Autodesk Inventor part; units mm, degrees
ref_plane "YZ Plane" through (0, 0, 0) normal (1, 0, 0) x (0, 1, 0)
ref_plane "XZ Plane" through (0, 0, 0) normal (0, 1, 0) x (-1, 0, 0)
ref_plane "XY Plane" through (0, 0, 0) normal (0, 0, 1) x (1, 0, 0)
sketch "Szkic1" plane through (0, 0, 0) normal (0, 0, 1) x (1, 0, 0)
  line L0 (-98.62, 58.242) -> (467.38, 58.242)
  line L1 (467.38, 58.242) -> (467.38, -3.758)
  line L2 (467.38, -3.758) -> (-98.62, -3.758)
  line L3 (-98.62, -3.758) -> (-98.62, 58.242)
  line L4 (65.48, 58.242) -> (95.48, 58.242)
  line L5 (95.48, 58.242) -> (95.48, 86.242)
  line L6 (95.48, 86.242) -> (65.48, 86.242)
  line L7 (65.48, 86.242) -> (65.48, 58.242)
  line L8 (258.28, 58.242) -> (288.28, 58.242)
  line L9 (288.28, 58.242) -> (288.28, 86.242)
  line L10 (288.28, 86.242) -> (258.28, 86.242)
  line L11 (258.28, 86.242) -> (258.28, 58.242)
  line L12 (-98.62, 58.242) -> (-98.62, 88.242)
  line L13 (-98.62, 88.242) -> (-68.62, 88.242)
  line L14 (-68.62, 88.242) -> (-68.62, 58.242)
  line L15 (-28.62, 50.242) -> (21.38, 50.242)
  line L16 (21.38, 50.242) -> (21.38, 0.242)
  line L17 (21.38, 0.242) -> (-28.62, 0.242)
  line L18 (-28.62, 0.242) -> (-28.62, 50.242)
  circle A0 centre (-23.62, 45.242) radius 1.5
  circle A1 centre (16.38, 45.242) radius 1.5
  circle A2 centre (-23.62, 5.242) radius 1.5
  circle A3 centre (16.38, 5.242) radius 1.5
  circle A4 centre (-3.62, 25.242) radius 24
  circle A5 centre (-3.62, 25.242) radius 11
  arc A6 (9.6779, 5.2628) -> (4.7367, 18.0889) centre (-10.3192, 4.9238) ccw
  arc A7 (12.5064, 7.4673) -> (6.6011, 21.1764) centre (-7.4877, 6.9811) ccw
  arc A8 (19.4906, 31.7151) -> (5.7653, 30.9792) centre (13.6335, 12.592) ccw
  arc A9 (18.2681, 35.0864) -> (3.4051, 33.7065) centre (12.552, 15.9207) ccw
  arc A10 (-2.6348, 49.2217) -> (-6.1762, 35.9408) centre (13.7425, 37.742) ccw
  arc A11 (-6.2188, 49.1008) -> (-9.4993, 34.5389) centre (10.2425, 37.742) ccw
  arc A12 (-26.1217, 33.5891) -> (-14.5851, 26.117) centre (-10.1429, 45.6174) ccw
  arc A13 (-27.1142, 30.1431) -> (-14.2787, 22.5233) centre (-11.2244, 42.2887) ccw
  arc A14 (-18.512, 6.421) -> (-7.8406, 15.0839) centre (-25.0139, 25.3347) ccw
  arc A15 (-15.5414, 4.4122) -> (-4.3281, 14.2648) centre (-22.1823, 23.2774) ccw
  line L19 (36.38, 50.242) -> (86.38, 50.242)
  line L20 (86.38, 50.242) -> (86.38, 0.242)
  line L21 (86.38, 0.242) -> (36.38, 0.242)
  line L22 (36.38, 0.242) -> (36.38, 50.242)
  circle A16 centre (41.38, 45.242) radius 1.5
  circle A17 centre (81.38, 45.242) radius 1.5
  circle A18 centre (41.38, 5.242) radius 1.5
  circle A19 centre (81.38, 5.242) radius 1.5
  circle A20 centre (61.38, 25.242) radius 24
  circle A21 centre (61.38, 25.242) radius 11
  arc A22 (74.6779, 5.2628) -> (69.7367, 18.0889) centre (54.6808, 4.9238) ccw
  arc A23 (77.5064, 7.4673) -> (71.6011, 21.1764) centre (57.5123, 6.9811) ccw
  arc A24 (84.4906, 31.7151) -> (70.7653, 30.9792) centre (78.6335, 12.592) ccw
  arc A25 (83.2681, 35.0864) -> (68.4051, 33.7065) centre (77.552, 15.9207) ccw
  arc A26 (62.3652, 49.2217) -> (58.8238, 35.9408) centre (78.7425, 37.742) ccw
  arc A27 (58.7812, 49.1008) -> (55.5007, 34.5389) centre (75.2425, 37.742) ccw
  arc A28 (38.8783, 33.5891) -> (50.4149, 26.117) centre (54.8571, 45.6174) ccw
  arc A29 (37.8858, 30.1431) -> (50.7213, 22.5233) centre (53.7756, 42.2887) ccw
  arc A30 (46.488, 6.421) -> (57.1594, 15.0839) centre (39.9861, 25.3347) ccw
  arc A31 (49.4586, 4.4122) -> (60.6719, 14.2648) centre (42.8177, 23.2774) ccw
  point P0 (0, 0)
  point P1 (80.48, 71.242)
  point P2 (273.28, 71.242)
  point P3 (-81.62, 68.242)
  point P4 (450.38, 43.242)
  point P5 (-81.62, 11.242)
  point P6 (450.38, 11.242)
  dimension "d0" = 566
  dimension "d1" = 62
  dimension "d2" = 30
  dimension "d3" = 28
  dimension "d4" = 30
  dimension "d5" = 28
  dimension "d6" = 164.1
  dimension "d7" = 356.9
  dimension "d11" = 17
  dimension "d12" = 17
  dimension "d13" = 15
  dimension "d14" = 15
  dimension "d15" = 15
  dimension "d16" = 15
  dimension "d18" = 15
  dimension "d26" = 17
  dimension "d27" = 17
  dimension "d28" = 15
  dimension "d29" = 15
  dimension "d30" = 30
  dimension "d31" = 30
  dimension "d36" = 20
  dimension "d38" = 50
  dimension "d39" = 50
  dimension "d42" = 8
  dimension "d44" = 70
  dimension "d46" = 5
  dimension "d47" = 5
  dimension "d48" = 5
  dimension "d49" = 5
  dimension "d50" = 5
  dimension "d51" = 5
  dimension "d52" = 5
  dimension "d53" = 5
  dimension "d54" = 3
  dimension "d55" = 3
  dimension "d56" = 3
  dimension "d92" = 25
  dimension "d98" = 25
  dimension "d99" = 50
  dimension "d100" = 50
  dimension "d101" = 5
  dimension "d102" = 5
  dimension "d103" = 5
  dimension "d104" = 5
  dimension "d105" = 5
  dimension "d106" = 5
  dimension "d107" = 5
  dimension "d108" = 5
  dimension "d109" = 3
  dimension "d110" = 3
  dimension "d111" = 3
  dimension "d112" = 25
  dimension "d113" = 25
  dimension "d114" = 15
  dimension "d115" = 8
extrude "Wyciągnięcie proste1" add sketch "Szkic1" along normal blind 2 contours L12 L13 L14 L0 | L0 L1 L2 L3 | L7 L6 L5 L0 | L11 L10 L9 L0 | L15 L16 L17 L18 | A0 | A1 | A2 | A3 | A4 A7 A5 A8 | A8 A5 A9 A4 | A4 A6 A5 A7 | A9 A5 A10 A4 | A5 | A4 A15 A5 A6 | A10 A5 A11 A4 | A4 A14 A5 A15 | A11 A5 A12 A4 | A4 A13 A5 A14 | A12 A5 A13 A4 | L19 L20 L21 L22 | A16 | A17 | A18 | A19 | A20 A23 A21 A24 | A24 A21 A25 A20 | A20 A22 A21 A23 | A25 A21 A26 A20 | A21 | A20 A31 A21 A22 | A26 A21 A27 A20 | A20 A30 A21 A31 | A27 A21 A28 A20 | A20 A29 A21 A30 | A28 A21 A29 A20
fillet "Zaokrąglenie1" radius 10 8 edges at (95.48, 86.242, 1) (95.48, 58.242, 1) (65.48, 58.242, 1) (65.48, 86.242, 1) (258.28, 58.242, 1) (258.28, 86.242, 1) (288.28, 86.242, 1) (288.28, 58.242, 1)
hole "Otwór1" at (80.48, 71.242, 0) at (273.28, 71.242, 0) at (-81.62, 68.242, 0) at (450.38, 43.242, 0) at (-81.62, 11.242, 0) at (450.38, 11.242, 0) direction (0, 0, 1) diameter 4 end through all
fillet "Zaokrąglenie3" radius 30 2 edges at (-68.62, 58.242, 1) (-68.62, 88.242, 1)
extrude "Wyciągnięcie proste3" cut sketch "Szkic1" along normal through all contours A0 | A1 | A2 | A3 | A4 A7 A5 A8 | A9 A5 A10 A4 | A4 A15 A5 A6 | A11 A5 A12 A4 | A4 A13 A5 A14 | A16 | A17 | A18 | A19 | A20 A23 A21 A24 | A25 A21 A26 A20 | A20 A31 A21 A22 | A27 A21 A28 A20 | A20 A29 A21 A30
properties part number "LC_ALU_2mm_Left_Plate"
Check sheet for the modelled part. Datum: model origin and axes. Units: mm. A direction names the side the tool comes from. Give positions to 0.01 mm unless a question says otherwise; leave off trailing zeros. Loops run counter-clockwise (first coordinate to the right, second up) from the corner with the lowest first, then second, coordinate; pieces in that order, holes last. Notation, with made-up numbers: M 86.25,-35 L 111.25,-35 A25 ccw 111.25,-9 Z; hole C -28,-37.5 d6. An arc over 180 degrees is marked long. Answer as a JSON object with one key per item and string values. Group by question number.
Q1. Cross-section at A-A on x = 30. Record the cut outline in (y, z).
Q2. Cross-section at B-B on z = 1.45. Give the number of separate pieces and of enclosed holes in the cut face, then the cut area to 3 significant figures.
Q3. Release check for a two-part mould opening along X. For faces 1 (the flat face through (180, 33, 0)), 2 (the cylindrical face through (74.67, 45.227, 0.986)), 3 (the cylindrical face through (285.428, 83.235, 1.014)) record: released by +X, released by -X, zero draft, split by the parting line, or undercut.
Q4. Material ranges on line 1 along Y through (x, z) = (-23.62, 1.5); line 2 along X through (y, z) = (3.5, 1.75); line 3 along Y through (x, z) = (82, 1.3), recorded low to high. Write a range as [from, to].
Q5. Access from +Z, -Z, +X, -X, +Y, -Y to the whole of each face (thin tool, end or side, straight path). Record for faces 4 (the flat face through (180, 33, 2)), 5 (the cylindrical face through (-53.81, 62.37, 1.01)).
Q6. Go/stop test with flat-tipped pins: P1, Ø1, axis at x = 78.5, z = 0.5, coming from the +Y side; P2, Ø1, axis at x = -19, z = 2, coming from the +Y side. Record where each tip stops, or that it passes through.
Evaluation:
{
 "1": {"outline": "M -3.76,0 L 58.24,0 L 58.24,2 L -3.76,2 Z"},
 "2": {"separate pieces": "1", "enclosed holes": "24", "area": "35,300 mm2"},
 "3": {"face 1": "zero draft", "face 2": "undercut", "face 3": "released by +X"},
 "4": {"line 1": "y = [-3.76, 3.74], [6.74, 11.98], [26.59, 30.84], [38.51, 43.74], [46.74, 58.24]", "line 2": "x = [-98.62, -13.78], [6.54, 51.22], [71.54, 467.38]", "line 3": "y = [-3.76, 3.88], [6.61, 12.96], [32.31, 35.42], [37.52, 43.88], [46.61, 69.94], [72.54, 86.24]"},
 "5": {"face 4": "+Z, +X, -X, +Y, -Y", "face 5": "+Z, -Z, +Y"},
 "6": {"P1": "stops at y = 86.24", "P2": "stops at y = 58.24"}
}
